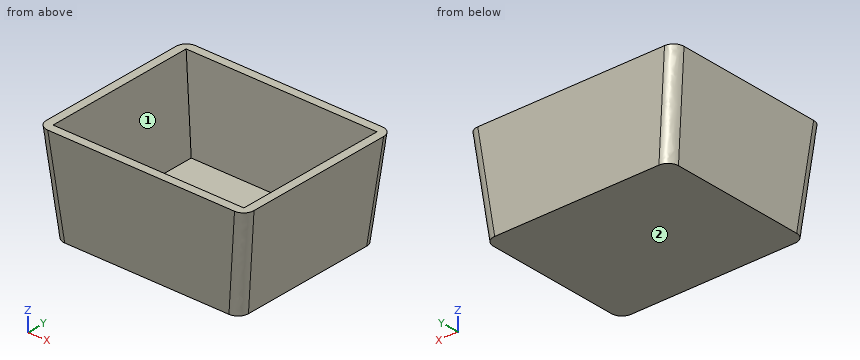
from build123d import *

# Parameters (mm, degrees)
F2_W = 17.7
F2_H = 14.95
F4_W = 19.85
F4_H = 16.2
F6_T = -0.8
F7_R = 1


with BuildPart() as f5:
    # F2 (on Top) → F5 section 0
    with BuildSketch(Plane.XY):
        with Locations((-241.6565716267, 110.767347253)):
            Rectangle(F2_W, F2_H)
    # F4 (on offset) → F5 section 1
    with BuildSketch(Plane.XY.offset(9.25)):
        with Locations((-241.6565716267, 110.767347253)):
            Rectangle(F4_W, F4_H)
    loft()

    # F6
    f6_openings = [f5.faces().sort_by_distance(p)[0] for p in [
        (-241.656572, 110.767347, 9.25),
    ]]
    offset(amount=F6_T, openings=f6_openings)

    # F7
    f7_edges = [f5.edges().sort_by_distance(p)[0] for p in [
        (-251.044072, 102.979847, 4.625),
        (-232.269072, 102.979847, 4.625),
        (-232.269072, 118.554847, 4.625),
        (-251.044072, 118.554847, 4.625),
    ]]
    fillet(f7_edges, radius=F7_R)


solid = f5.part
Can you work these out from the model? Positions are in its coordinate system, mm. Face numbers are marked on the shaded views. Give positions to 0.01 mm unless a question says otherwise; leave off trailing zeros. Use a Markdown table: item, result. Add a question column.
Item 1: Will these pins go through, and if not, where does the flat tip stop? pin 1 (3 mm diameter, centred on y = 112.5, z = 3.5, fed in from +X); pin 2 (2 mm diameter, centred on y = 111, z = 7, fed in from +X); pin 3 (3 mm diameter, centred on y = 110, z = 1.5, fed in from -X).
Item 2: If I drill on L1, parallel to Z at x = -238, y = 112.75; L2, parallel to X at y = 111.5, z = 1.25; L3, parallel to X at y = 106.5, z = 7, over which ranges is the centre line in solid material (lowest first)? Write a range as [from, to].
Item 3: We'd pull the mould along X, two halves only. Please class the marked faces 1 and 2: +X half, -X half, draft (parallel to the pull), parting line (faces both ways), or undercut.
Answer sheet:
| question | item | result |
|---|---|---|
| 1 | pin 1 | stops at x = -232.23 |
| 1 | pin 2 | stops at x = -231.88 |
| 1 | pin 3 | stops at x = -250.86 |
| 2 | L1 | z = [0, 0.8] |
| 2 | L2 | x = [-250.65, -249.85], [-233.47, -232.66] |
| 2 | L3 | x = [-251.32, -250.51], [-232.8, -231.99] |
| 3 | face 1 | undercut |
| 3 | face 2 | draft |
